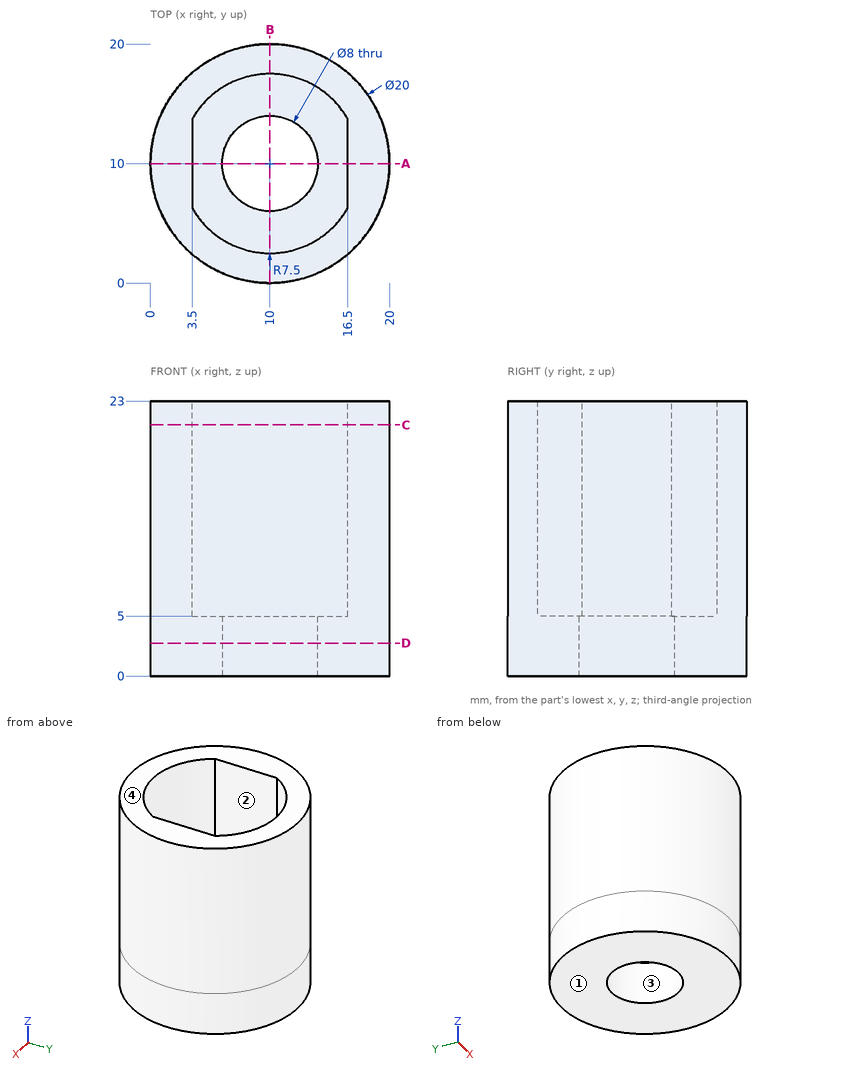
Geometry check sheet. Reference: drawing and pictorial views, mm from the part's lowest x, y, z. A direction names the side the tool comes from. Round coordinates to 2 decimals unless told otherwise and drop trailing zeros. Write each loop counter-clockwise with the first axis right and the second up, starting at its lowest first coordinate (ties: lowest second). Pieces come first, ordered by that corner, then holes.
1. Draft check along Y on the marked faces 3 and 4. Enter one of: +Y half, -Y half, draft (parallel to the pull), parting line (faces both ways), or undercut.
2. Section check A-A on y = 10. Enter the section's corners in (x, z).
3. Scan lines: L1, parallel to Y at x = 10, z = 3.8; L2, parallel to Z at x = 11, y = 5.25; L3, parallel to Y at x = 12.5, z = 2.75. Record each from-to range of solid material in increasing order.
4. Section check D-D on z = 2.75. Enter the section's corners in (x, y).
5. Gauge pin test, flat ends, axial feed: P1, Ø9, axis at x = 10, y = 10, coming from the +Z side; P2, Ø8, axis at y = 9.5, z = 5, coming from the +X side; P3, Ø10, axis at y = 16.5, z = 9.5, coming from the -X side; P4, Ø5, axis at y = 6.5, z = 7.5, coming from the +X side. Record the tip position at first contact, or that the pin passes through.
6. Section check C-C on z = 21. Enter the section's corners in (x, y).
7. Section check B-B on x = 10. Enter the section's corners in (y, z).
8. Access from +Z, -Z, +X, -X, +Y, -Y to the whole of each face (thin tool, end or side, straight path). Record for the marked faces 1 and 2.
Answer:
1. face 3: undercut
1. face 4: draft
2. outline: (0, 0) - (6, 0) - (6, 5) - (3.5, 5) - (3.5, 23) - (0, 23) - close; (14, 0) - (20, 0) - (20, 23) - (16.5, 23) - (16.5, 5) - (14, 5) - close
3. L1: y = 0 to 6, 14 to 20
3. L2: z = 0 to 5
3. L3: y = 0.32 to 6.88, 13.12 to 19.68
4. outline: circle Ø20 at (10, 10); hole circle Ø8 at (10, 10)
5. P1: stops at z = 5
5. P2: stops at x = 20
5. P3: stops at x = 0.11
5. P4: stops at x = 19.95
6. outline: circle Ø20 at (10, 10); hole (3.5, 6.26) arc R7.5 ccw to (16.5, 6.26) - (16.5, 13.74) arc R7.5 ccw to (3.5, 13.74) - close
7. outline: (0, 0) - (6, 0) - (6, 5) - (2.5, 5) - (2.5, 23) - (0, 23) - close; (14, 0) - (20, 0) - (20, 23) - (17.5, 23) - (17.5, 5) - (14, 5) - close
8. face 1: -Z, +X, -X, +Y, -Y
8. face 2: +Z
